Autodesk Inventor part; units mm, degrees
ref_plane "YZ Plane" through (0, 0, 0) normal (1, 0, 0) x (0, 1, 0)
ref_plane "XZ Plane" through (0, 0, 0) normal (0, 1, 0) x (-1, 0, 0)
ref_plane "XY Plane" through (0, 0, 0) normal (0, 0, 1) x (1, 0, 0)
sketch "スケッチ1" plane through (0, 0, 0) normal (0, 1, 0) x (-1, 0, 0)
  line L0 (56, 20) -> (-56, 20)
  line L1 (-56, 20) -> (-56, -20)
  line L2 (-56, -20) -> (56, -20)
  line L3 (56, -20) -> (56, 20)
  line L4 (56, 20) -> (-56, -20) construction
  line L5 (-56, 20) -> (56, -20) construction
  point P0 (0, 0)
  dimension "d0" = 112
  dimension "d1" = 40
extrude "押し出し1" add sketch "スケッチ1" along normal blind 10
sketch "スケッチ2" plane through (0, 10, 0) normal (0, 1, 0) x (1, 0, 0)
  line L0 (56, 20) -> (-56, 20)
  line L1 (-56, -20) -> (56, -20)
  line L2 (-56, 20) -> (4, 20)
  line L3 (4, 20) -> (4, -20)
  line L4 (4, -20) -> (-56, -20)
  line L5 (-56, -20) -> (-56, 20)
  line L6 (56, -20) -> (56, 20)
  line L7 (56, 20) -> (8, 20)
  line L8 (8, 20) -> (8, -20)
  line L9 (8, -20) -> (56, -20)
  line L10 (56, -20) -> (56, 20)
  point P0 (0, 0)
  point P1 (-56, -20)
  point P2 (4, 20)
  point P3 (8, 20)
  dimension "d4" = 60
  dimension "d5" = 48
extrude "押し出し2" cut sketch "スケッチ2" against normal blind 6 contours L6 L1 L8 L0 | L3 L1 L5 L0
fillet "フィレット1" radius 2 4 edges at (-56, 2, 20) (-56, 2, -20) (56, 2, -20) (56, 2, 20)
sketch "スケッチ3" plane through (0, 4, 0) normal (0, 1, 0) x (1, 0, 0)
  line L0 (-51, -15) -> (-1, -15)
  line L1 (-1, -15) -> (-1, 15)
  line L2 (-1, 15) -> (-51, 15)
  line L3 (-51, 15) -> (-51, -15)
  line L4 (-51, -15) -> (-1, 15) construction
  line L5 (-1, -15) -> (-51, 15) construction
  line L6 (13, -15) -> (51, -15)
  line L7 (51, -15) -> (51, 15)
  line L8 (51, 15) -> (13, 15)
  line L9 (13, 15) -> (13, -15)
  line L10 (13, -15) -> (51, 15) construction
  line L11 (51, -15) -> (13, 15) construction
  line L12 (8, 20) -> (54, 20)
  line L13 (56, 18) -> (56, -18)
  line L14 (54, -20) -> (8, -20)
  line L15 (8, -20) -> (8, 20)
  line L16 (-54, 20) -> (4, 20)
  line L17 (-56, -18) -> (-56, 18)
  line L18 (4, -20) -> (-54, -20)
  line L19 (4, 20) -> (4, -20)
  point P0 (0, 0)
  point P1 (-26, 0)
  point P2 (32, 0)
  dimension "d9" = 5
  dimension "d10" = 5
  dimension "d11" = 5
  dimension "d12" = 5
  dimension "d13" = 5
  dimension "d14" = 5
  dimension "d15" = 5
  dimension "d16" = 5
extrude "押し出し3" cut sketch "スケッチ3" against normal blind 6
fillet "フィレット2" radius 2 8 edges at (-51, 2, -15) (-1, 2, -15) (-51, 2, 15) (-1, 2, 15) (13, 2, -15) (51, 2, -15) (13, 2, 15) (51, 2, 15)
equation "\"d10\" = d9"
equation "\"d11\" = d9"
equation "\"d12\" = d9"
equation "\"d13\" = d9"
equation "\"d14\" = d9"
equation "\"d15\" = d9"
equation "\"d16\" = d9"
For this review, take the finished solid that the model builds, in its own axes (mm). A direction names the side the tool comes from. Coordinates: 2 decimals unless noted, no trailing zeros. Order: outer loops, then holes, each group sorted by start corner. A loop starts at its lowest first (then second) coordinate and runs counter-clockwise, first axis right, second up. Notation, with made-up numbers: (78, -13) - (87, -13) arc R16 cw to (87, -6) - close; hole circle Ø11 at (77, -30). An arc over 180 degrees is marked (long way). Answer as CSV lines item,"result". Start each with the question number.
1) Insertion check: P1, Ø1.5, axis at y = 6, z = -8, coming from the -X side; P2, Ø5, axis at x = 17.5, z = -3.5, coming from the -Y side; P3, Ø4, axis at x = -31.5, z = -14, coming from the +Y side; P4, Ø1.8, axis at y = 7, z = -6, coming from the +X side. Each pin has a flat end and moves straight along its axis. Give the tip position at first contact, or say it passes through.
2) Machinability: for faces 5 (the flat face through (-26, 4, 17)), 6 (the flat face through (8, 7, 0)), 7 (the flat face through (-1, 2, 20)), 8 (the flat face through (-26, 2, -15)), which of the approach directions +Z, -Z, +X, -X, +Y, -Y give a long, thin tool a straight path to every point of the face, cutting with its end or side? Answer none if there is none.
3) Add section C-C (y = 2.5). State the section outline as (x, z) points, then the cut area to 3 significant figures.
4) Draft analysis for pull direction X (two halves, no side actions). For faces 1 (the flat face through (51, 2, 0)), 2 (the cylindrical face through (-55.4, 2.03, -19.43)), 3 (the cylindrical face through (13.6, 1.97, 14.43)), 4 (the flat face through (56, 2, 0)), state which applies: +X half, -X half, draft (parallel to the pull), parting line (faces both ways), or undercut.
5) Add section B-B (z = 4). State the section outline as (x, y) points.
6) Add section D-D (y = 9). State the section outline as (x, z) points, then the cut area to 3 significant figures.
7) Add section A-A (x = 26.5). State the section outline as (y, z) points.
8) To check wall thickness, follow line 1 along X through (y, z) = (3.75, 12.5); line 2 along Z through (x, y) = (-39, 1.5); line 3 along X through (y, z) = (6.75, 8). State the ranges of each line that lie inside material, in increasing order. Write a range as [from, to].
Result:
1,P1,"x = 4"
1,P2,"through"
1,P3,"y = 4"
1,P4,"x = 8"
2,face 5,"+Z, -Z, -X, +Y"
2,face 6,"+Z, -Z, +X, +Y"
2,face 7,"+Z, +X, -X, +Y, -Y"
2,face 8,"+Y, -Y"
3,outline,"(-56, -18) arc R2 ccw to (-54, -20) - (54, -20) arc R2 ccw to (56, -18) - (56, 18) arc R2 ccw to (54, 20) - (-54, 20) arc R2 ccw to (-56, 18) - close; hole (-51, -13) arc R2 ccw to (-49, -15) - (-3, -15) arc R2 ccw to (-1, -13) - (-1, 13) arc R2 ccw to (-3, 15) - (-49, 15) arc R2 ccw to (-51, 13) - close; hole (13, -13) arc R2 ccw to (15, -15) - (49, -15) arc R2 ccw to (51, -13) - (51, 13) arc R2 ccw to (49, 15) - (15, 15) arc R2 ccw to (13, 13) - close"
3,area,"1,840 mm^2"
4,face 1,"undercut"
4,face 2,"-X half"
4,face 3,"undercut"
4,face 4,"+X half"
5,outline,"(-56, 0) - (-51, 0) - (-51, 4) - (-56, 4) - close; (-1, 0) - (13, 0) - (13, 4) - (8, 4) - (8, 10) - (4, 10) - (4, 4) - (-1, 4) - close; (51, 0) - (56, 0) - (56, 4) - (51, 4) - close"
6,outline,"(4, -20) - (8, -20) - (8, 20) - (4, 20) - close"
6,area,"160 mm^2"
7,outline,"(0, -20) - (4, -20) - (4, -15) - (0, -15) - close; (0, 15) - (4, 15) - (4, 20) - (0, 20) - close"
8,line 1,"[-56, -51], [-1, 13], [51, 56]"
8,line 2,"[-20, -15], [15, 20]"
8,line 3,"[4, 8]"
